Read the model definition and answer for the solid it produces. Units are mm, in the model's axes. Face numbers are marked on the shaded views. A direction names the side the tool comes from. Give positions to 0.01 mm unless a question says otherwise; leave off trailing zeros. Write each loop counter-clockwise with the first axis right and the second up, starting at its lowest first coordinate (ties: lowest second). Pieces come first, ordered by that corner, then holes. Notation, with made-up numbers: (71, 14.25) -> (127, 14.25) arc R18 cw to (127, 30.25) -> close; hole circle Ø10 at (15, 64). An arc over 180 degrees is marked (long way). Use a Markdown table: item, result.
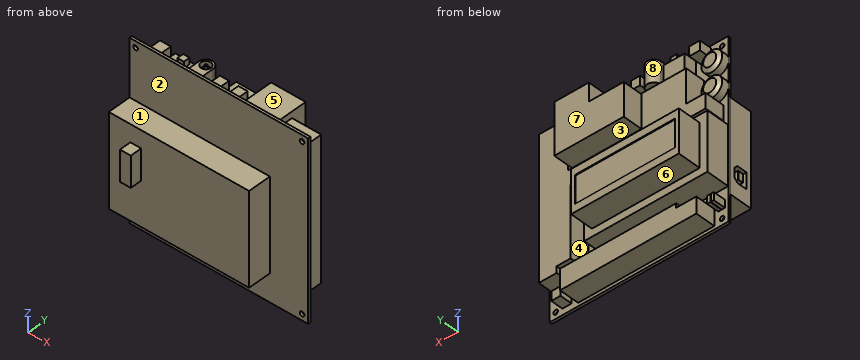
from build123d import *
from OCP.BRepFilletAPI import BRepFilletAPI_MakeChamfer

# Parameters (mm, degrees)
SKETCH1_W              = 116
SKETCH1_H              = 115
SKETCH1_R              = 1.5
BASE_FLANGE1_DEPTH     = 1.65
SKETCH3_W              = 79.9
SKETCH3_H              = 38
EXTRUDE1_DEPTH         = 15
SKETCH4_W              = 69.9
SKETCH4_H              = 28
EXTRUDE2_DEPTH         = 15
SKETCH6_W              = 64.9
SKETCH6_H              = 18
DISPLAY_DEPTH          = 0.53
SKETCH7_W              = 91
SKETCH7_H              = 60
WIRING_BOARD_DEPTH     = 15
SKETCH8_W              = 7
SKETCH8_H              = 20
EXTRUDE5_DEPTH         = 7.5
SKETCH9_W              = 10.5
SKETCH9_H              = 8.5
SKETCH9_W_2            = 5.5
SKETCH9_H_2            = 3.5
USB_DEPTH              = 7.5
CHAMFER1_SIZE          = 2
SKETCH10_R             = 6.75
POTENTIOMETERS_DEPTH   = 6.2
SKETCH11_W             = 7
SKETCH11_H             = 6.1
SKETCH11_W_2           = 9
SKETCH11_H_2           = 14.3
SKETCH11_W_3           = 6
SKETCH11_H_3           = 6
SKETCH11_W_4           = 2
SKETCH11_H_4           = 5
KEEP_ACCESSIBLE_DEPTH  = 8
EXTRUDE9_DEPTH         = 13
HOT_VOLTAGE_REGS_DEPTH = 23.5
SKETCH14_R             = 4.5
EXTRUDE10_DEPTH        = 14.3
EXTRUDE11_DEPTH        = 10
EXTRUDE11_DEPTH_BACK   = 3.4
SKETCH15_R             = 3.219788924
SKETCH15_R_2           = 0.896300673
SKETCH15_W             = 5.949829442
SKETCH15_H             = 2.638553101
SKETCH15_H_2           = 2.133019186
FILLET1_R              = 0.2
CHAMFER2_SIZE          = 1.5
CHAMFER2_SIZE2         = 2.5


# Sheet-metal steps are written as plain solids
with BuildPart() as part:
    # Sketch1 → Base-Flange1 (new body)
    with BuildSketch(Plane(origin=(0, 0, 0), x_dir=(1, 0, 0), z_dir=(0, 1, 0))):
        Rectangle(SKETCH1_W, SKETCH1_H)
        with Locations(Location((54, 53.4, 0), (0, 0, 270))):
            Circle(SKETCH1_R, mode=Mode.SUBTRACT)
        with Locations(Location((54, -53.4, 0), (0, 0, 90))):
            Circle(SKETCH1_R, mode=Mode.SUBTRACT)
        with Locations(Location((-54, 53.4, 0), (0, 0, 90))):
            Circle(SKETCH1_R, mode=Mode.SUBTRACT)
        with Locations(Location((-54, -53.4, 0), (0, 0, 270))):
            Circle(SKETCH1_R, mode=Mode.SUBTRACT)
    extrude(amount=BASE_FLANGE1_DEPTH)

    # Sketch3 → Extrude1 (add)
    with BuildSketch(Plane(origin=(0, 1.65, 0), x_dir=(1, 0, 0), z_dir=(0, 1, 0))):
        with Locations((-17.95, 16.5)):
            Rectangle(SKETCH3_W, SKETCH3_H)
    extrude(amount=EXTRUDE1_DEPTH)

    # Sketch4 → Extrude2 (add)
    with BuildSketch(Plane(origin=(0, 16.65, 0), x_dir=(1, 0, 0), z_dir=(0, 1, 0))):
        with Locations((-17.95, 16.5)):
            Rectangle(SKETCH4_W, SKETCH4_H)
    extrude(amount=EXTRUDE2_DEPTH)

    # Sketch6 → Display! (cut)
    with BuildSketch(Plane(origin=(0, 31.65, 0), x_dir=(1, 0, 0), z_dir=(0, 1, 0))):
        with Locations((-17.95, 16.5)):
            Rectangle(SKETCH6_W, SKETCH6_H)
    extrude(amount=-DISPLAY_DEPTH, mode=Mode.SUBTRACT)

    # Sketch7 → Wiring Board (add)
    with BuildSketch(Plane.XZ):
        with Locations((-12.4, -9.5)):
            Rectangle(SKETCH7_W, SKETCH7_H)
    extrude(amount=WIRING_BOARD_DEPTH)

    # Sketch8 → Extrude5 (add)
    with BuildSketch(Plane.XZ.offset(15)):
        with Locations((-40.4, -0.8)):
            Rectangle(SKETCH8_W, SKETCH8_H)
    extrude(amount=EXTRUDE5_DEPTH)

    # Sketch9 → USB (cut)
    with BuildSketch(Plane.ZY.offset(58)):
        with Locations((-24.25, -7.35)):
            Rectangle(SKETCH9_W, SKETCH9_H)
        with Locations((-24.25, -7.35)):
            Rectangle(SKETCH9_W_2, SKETCH9_H_2, mode=Mode.SUBTRACT)
    extrude(amount=-USB_DEPTH, mode=Mode.SUBTRACT)

    # Chamfer1
    chamfer1_edges = [part.edges().sort_by_distance(p)[0] for p in [
        (-54.2, -3.1, -19),
        (-54.2, -3.1, -29.5),
    ]]
    chamfer(chamfer1_edges, length=CHAMFER1_SIZE)

    # Sketch10 → Potentiometers (add)
    with BuildSketch(Plane(origin=(0, 1.65, 0), x_dir=(1, 0, 0), z_dir=(0, 1, 0))):
        with Locations(Location((-51.5, -26.5, 0), (0, 0, 164.357528987))):
            Circle(SKETCH10_R)
        with Locations(Location((-51.5, -42.5, 0), (0, 0, 164.357528987))):
            Circle(SKETCH10_R)
    extrude(amount=POTENTIOMETERS_DEPTH)

    # Sketch11 → Keep Accessible!! (add)
    with BuildSketch(Plane(origin=(0, 1.65, 0), x_dir=(1, 0, 0), z_dir=(0, 1, 0))):
        Polygon((-26.092034571, -53.3), (-23.1, -53.3), (-23.1, -42.3), (-36.9, -42.3), (-36.9, -53.3), (-30.292034571, -53.3), (-30.292034571, -57.5), (-26.092034571, -57.5), align=None)
        with Locations((-43.3, -52.95)):
            Rectangle(SKETCH11_W, SKETCH11_H)
        with Locations((-17, -49.55)):
            Rectangle(SKETCH11_W_2, SKETCH11_H_2)
        with Locations((-5, -52.1)):
            Rectangle(SKETCH11_W_3, SKETCH11_H_3)
        with Locations((7, -52.1)):
            Rectangle(SKETCH11_W_3, SKETCH11_H_3)
        with Locations((46.66, 50.5)):
            Rectangle(SKETCH11_W_3, SKETCH11_H_3)
        with Locations((-54.82, 45.3)):
            Rectangle(SKETCH11_W_4, SKETCH11_H_4)
        with Locations((-52.52, 45.3)):
            Rectangle(SKETCH11_W_4, SKETCH11_H_4)
    extrude(amount=KEEP_ACCESSIBLE_DEPTH)

    # Sketch12 → Extrude9 (add)
    with BuildSketch(Plane(origin=(0, 1.65, 0), x_dir=(1, 0, 0), z_dir=(0, 1, 0))):
        Polygon((-48.948570669, 53.670290093), (-48.948570669, 44.832154672), (-35.833918109, 44.832154672), (-35.833918109, 41.981143246), (37.294524965, 41.981143246), (39.432783534, 41.981143246), (39.432783534, 53.670290093), (39.432783534, 55.380896948), (-48.948570669, 55.380896948), align=None)
        Polygon((41.713592675, 43.406648959), (41.713592675, 39.272682392), (32.590356112, 39.272682392), (32.590356112, -6.486050994), (-54.935694663, -6.486050994), (-54.935694663, -16.179489842), (-42.391244389, -16.179489842), (-42.391244389, -38.132277821), (-13.310927845, -38.132277821), (-13.310927845, -16.179489842), (34.300962968, -16.179489842), (34.300962968, -48.538469526), (53.26018895, -48.538469526), (53.26018895, 43.406648959), align=None)
    extrude(amount=EXTRUDE9_DEPTH)

    # Sketch13 → Hot! Voltage Regs (add)
    with BuildSketch(Plane(origin=(0, 1.65, 0), x_dir=(1, 0, 0), z_dir=(0, 1, 0))):
        Polygon((-11.315219847, -18.602849554), (-11.315219847, -40.12798582), (11.350320989, -40.12798582), (11.350320989, -51.959683237), (33.730760683, -51.959683237), (33.730760683, -18.602849554), align=None)
    extrude(amount=HOT_VOLTAGE_REGS_DEPTH)

    # Sketch14 → Extrude10 (add)
    with BuildSketch(Plane.XY.offset(56.7)):
        with Locations((-17, 9.65)):
            Circle(SKETCH14_R)
    extrude(amount=-EXTRUDE10_DEPTH)

    # Sketch15 → Extrude11 (cut, two sides: drawn at the far end of the back side and taken through both)
    # profile 1 of 3: a face of its own
    with BuildSketch(Plane.XY.offset(56.7).offset(-EXTRUDE11_DEPTH_BACK)):
        with Locations(Location((-17, 9.65, 0), (0, 0, 180))):
            Circle(SKETCH15_R)
        with Locations(Location((-17, 9.65, 0), (0, 0, 180))):
            Circle(SKETCH15_R_2, mode=Mode.SUBTRACT)
    # profile 2 of 3: a face of its own
    with BuildSketch(Plane.XY.offset(56.7).offset(-EXTRUDE11_DEPTH_BACK)):
        with Locations((-28.188847243, 9.227024123)):
            Rectangle(SKETCH15_W, SKETCH15_H)
    # profile 3 of 3: a face of its own
    with BuildSketch(Plane.XY.offset(56.7).offset(-EXTRUDE11_DEPTH_BACK)):
        with Locations((-28.188847243, 2.716509593)):
            Rectangle(SKETCH15_W, SKETCH15_H_2)
    extrude(amount=EXTRUDE11_DEPTH + EXTRUDE11_DEPTH_BACK, mode=Mode.SUBTRACT)

    # Fillet1
    fillet1_edges = [part.edges().sort_by_distance(p)[0] for p in [
        (-16.103699327, 9.65, 56.7),
        (-57.9, -9.1, -24.25),
        (-57.9, -7.35, -21.5),
        (-57.9, -5.6, -24.25),
        (-57.9, -7.35, -27),
    ]]
    fillet(fillet1_edges, radius=FILLET1_R)

    # Chamfer2: one chamfer whose edges measure the first distance from different faces: ONE call of the kernel's chamfer builder (chamfer() names one face for all edges)
    chamfer2_edges_1 = [part.edges().sort_by_distance(p)[0] for p in [
        (-45, 7.85, 28.320027472),
    ]]
    chamfer2_side_1 = [part.faces().sort_by_distance(p)[0] for p in [
        (-45, 4.75, 28.320027472),
    ]]
    chamfer2_edges_2 = [part.edges().sort_by_distance(p)[0] for p in [
        (-45, 7.85, 44.320027472),
    ]]
    chamfer2_side_2 = [part.faces().sort_by_distance(p)[0] for p in [
        (-45, 4.75, 44.320027472),
    ]]
    chamfer2 = BRepFilletAPI_MakeChamfer(part.part.solid().wrapped)
    for e in chamfer2_edges_1:
        chamfer2.Add(CHAMFER2_SIZE, CHAMFER2_SIZE2, e.wrapped, chamfer2_side_1[0].wrapped)  # the first distance lies on this face
    for e in chamfer2_edges_2:
        chamfer2.Add(CHAMFER2_SIZE, CHAMFER2_SIZE2, e.wrapped, chamfer2_side_2[0].wrapped)  # the first distance lies on this face
    add(Compound.cast(chamfer2.Shape()), mode=Mode.REPLACE)


solid = part.part
Item 1: A cutting plane is placed at C-C (z = 11). Give the vertices of the cut face in (x, y), then the cut area to 3 significant figures.
Return value:
| item | result |
|---|---|
| outline | (-58, 0) -> (-57.9, 0) -> (-57.9, -15) -> (33.1, -15) -> (33.1, 0) -> (58, 0) -> (58, 1.65) -> (53.26, 1.65) -> (53.26, 14.65) -> (-54.94, 14.65) -> (-54.94, 1.65) -> (-58, 1.65) -> close |
| area | 2,960 mm^2 |
Item 2: A tool of negligible diameter and unlimited length cuts with its end or side. For the marked faces 4, 5, 6, 7 and 8, from which of +Z, -Z, +X, -X, +Y, -Y can it reach the whole face along a straight path? Write none if from no direction.
Return value:
| item | result |
|---|---|
| face 4 | +Y |
| face 5 | +Z, +X, +Y |
| face 6 | -Z, +X, -X, +Y |
| face 7 | +Z, +X, -X, +Y |
| face 8 | +Z, +Y |
Item 3: A cutting plane is placed at A-A (y = 19.5). Give the vertices of the cut face in (x, z), then the cut area to 3 significant figures.
Return value:
| item | result |
|---|---|
| outline | (-52.9, -30.5) -> (17, -30.5) -> (17, -2.5) -> (-52.9, -2.5) -> close; (-11.32, 18.6) -> (33.73, 18.6) -> (33.73, 51.96) -> (11.35, 51.96) -> (11.35, 40.13) -> (-11.32, 40.13) -> close |
| area | 3,190 mm^2 |
Item 4: Straight lines are drawn through the part: line 1 along X through (y, z) = (2.5, 50); line 2 along X through (y, z) = (0.8, 53.4); line 3 along X through (y, z) = (12, 30.5). For each, find the intervals that lie inside material, in ascending order. Write a range as [from, to].
Return value:
| item | result |
|---|---|
| line 1 | [-46.8, -39.8], [-36.9, -23.1], [-21.5, -12.5], [-8, -2], [4, 10], [11.35, 33.73] |
| line 2 | [-58, -55.5], [-52.5, 52.5], [55.5, 58] |
| line 3 | [-42.39, -13.31], [-11.32, 33.73], [34.3, 53.26] |
Item 5: For a pull along Z with two mould halves and no side action, classify the marked faces 1, 2 and 3 as +Z half, -Z half, draft (parallel to the pull), parting line (faces both ways), or undercut.
Return value:
| item | result |
|---|---|
| face 1 | +Z half |
| face 2 | draft |
| face 3 | undercut |
Item 6: Each of these flat-tipped pins is pushed along its axis until it touches: P1, Ø3, axis at x = 18, y = 9.5, coming from the -Z side; P2, Ø2.5, axis at y = 7.5, z = -45, coming from the +X side; P3, Ø6.5, axis at x = -4, z = 51, coming from the +Y side. Where does it stop, or does it pass through?
Return value:
| item | result |
|---|---|
| P1 | z = -55.38 |
| P2 | x = 39.43 |
| P3 | y = 9.65 |
